Geometry: final body of the model. Coordinates: model frame, mm. Face numbers are marked on the shaded views. Give positions to 0.01 mm unless a question says otherwise; leave off trailing zeros. Write each loop counter-clockwise with the first axis right and the second up, starting at its lowest first coordinate (ties: lowest second). Pieces come first, ordered by that corner, then holes. Notation, with made-up numbers: (-15.75, 54.25) -> (30.25, 54.25) arc R19 ccw to (30.25, 64.25) -> close; hole circle Ø3 at (29.5, -11). An arc over 180 degrees is marked (long way). Answer as a JSON object with one key per item and string values.
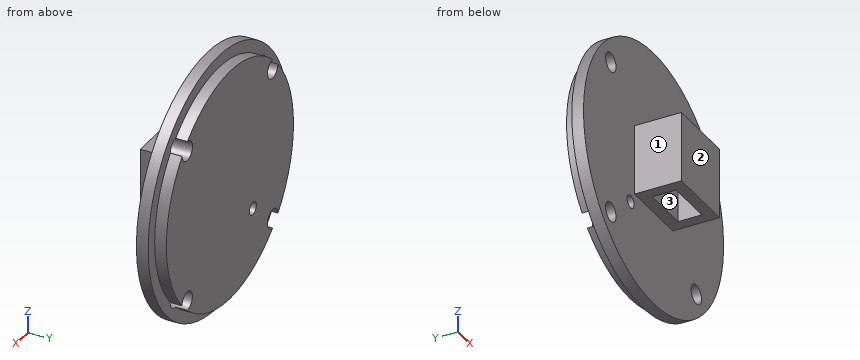
from build123d import *

# Parameters (mm, degrees)
SKETCH_1_R          = 55
EXTRUDE_1_DEPTH     = 5
SKETCH_2_R          = 49.9
EXTRUDE_2_DEPTH     = 5
SKETCH_3_W          = 30
SKETCH_3_H          = 30
EXTRUDE_3_DEPTH     = 20
SKETCH_4_W          = 20.2
SKETCH_4_H          = 10.2
CUT_EXTRUDE_1_DEPTH = 71
SKETCH_5_R          = 4.1
CUT_EXTRUDE_2_DEPTH = 11
SKETCH_6_R          = 2.75
CUT_EXTRUDE_3_DEPTH = 31


with BuildPart() as part:
    # Эскиз1 → Бобышка-Вытянуть1 (new body)
    with BuildSketch(Plane(origin=(0, 0, 0), x_dir=(1, 0, 0), z_dir=(0, 1, 0))):
        with Locations(Location((0, 0, 0), (0, 0, 270))):  # turned: the seam where the file's is
            Circle(SKETCH_1_R)
    extrude(amount=EXTRUDE_1_DEPTH)

    # Эскиз2 → Бобышка-Вытянуть2 (add)
    with BuildSketch(Plane(origin=(0, 5, 0), x_dir=(1, 0, 0), z_dir=(0, 1, 0))):
        with Locations(Location((0, 0, 0), (0, 0, 270))):  # turned: the seam where the file's is
            Circle(SKETCH_2_R)
    extrude(amount=EXTRUDE_2_DEPTH)

    # Эскиз3 → Бобышка-Вытянуть3 (add)
    with BuildSketch(Plane.XZ):
        Rectangle(SKETCH_3_W, SKETCH_3_H)
    extrude(amount=EXTRUDE_3_DEPTH)

    # Эскиз4 → Вырез-Вытянуть1 (cut, through all)
    with BuildSketch(Plane.XY.offset(15)):
        with Locations((0, -10)):
            Rectangle(SKETCH_4_W, SKETCH_4_H)
    extrude(amount=-CUT_EXTRUDE_1_DEPTH, mode=Mode.SUBTRACT)

    # Эскиз5 → Вырез-Вытянуть2 (cut, through all)
    with BuildSketch(Plane.XZ):
        with Locations(Location((33.592198598, -32.871936263, 0), (0, 0, 270))):  # turned: the seam where the file's is
            Circle(SKETCH_5_R)
        with Locations(Location((-33.591727056, -32.872418125, 0), (0, 0, 270))):  # turned: the seam where the file's is
            Circle(SKETCH_5_R)
        with Locations(Location((-33.591727056, 32.872418125, 0), (0, 0, 270))):  # turned: the seam where the file's is
            Circle(SKETCH_5_R)
        with Locations(Location((33.483215177, 32.983215177, 0), (0, 0, 270))):  # turned: the seam where the file's is
            Circle(SKETCH_5_R)
    extrude(amount=-CUT_EXTRUDE_2_DEPTH, mode=Mode.SUBTRACT)

    # Эскиз6 → Вырез-Вытянуть3 (cut, through all)
    with BuildSketch(Plane(origin=(0, 10, 0), x_dir=(1, 0, 0), z_dir=(0, 1, 0))):
        with Locations(Location((-17.999856554, 19.999999999, 0), (0, 0, 270))):  # turned: the seam where the file's is
            Circle(SKETCH_6_R)
    extrude(amount=-CUT_EXTRUDE_3_DEPTH, mode=Mode.SUBTRACT)


solid = part.part
Q1. Cut plane C-C (x = 0). Return the cut outline in (y, z), and give its area (3 significant figures).
Values:
{"outline": "(-20, -15) -> (-15.1, -15) -> (-15.1, 15) -> (-20, 15) -> close; (-4.9, -15) -> (0, -15) -> (0, -55) -> (5, -55) -> (5, -49.9) -> (10, -49.9) -> (10, 49.9) -> (5, 49.9) -> (5, 55) -> (0, 55) -> (0, 15) -> (-4.9, 15) -> close", "area": "1,340 mm²"}
Q2. First-contact query: P1, Ø6.5, axis at x = 33.59, z = -32.87, coming from the +Y side; P2, Ø3, axis at y = -10.5, z = 4, coming from the +X side; P3, Ø9, axis at x = -18, z = -20, coming from the +Y side; P4, Ø1.5, axis at x = -13, y = -6, coming from the +Z side. Flat tips, straight axial feed; report the tip coordinate or a pass-through.
Values:
{"P1": "through", "P2": "x = 15", "P3": "y = 10", "P4": "z = 15"}
Q3. Cut plane A-A (z = 0). Return the cut outline in (x, y), and give its area (3 significant figures).
Values:
{"outline": "(-55, 0) -> (-15, 0) -> (-15, -20) -> (15, -20) -> (15, 0) -> (55, 0) -> (55, 5) -> (49.9, 5) -> (49.9, 10) -> (-49.9, 10) -> (-49.9, 5) -> (-55, 5) -> close; hole (-10.1, -15.1) -> (10.1, -15.1) -> (10.1, -4.9) -> (-10.1, -4.9) -> close", "area": "1,440 mm²"}
Q4. Material intervals for L1, parallel to Y at x = 4.5, z = -6; L2, parallel to Z at x = 37, y = 3.25; L3, parallel to X at y = -10, z = 14.5, sorted ascending. Write a range as from..to.
Values:
{"L1": "-20..-15.1, -4.9..10", "L2": "-40.69..-35.15, -30.59..30.88, 35.09..40.69", "L3": "-15..-10.1, 10.1..15"}
Q5. Cut plane D-D (z = -20). Return the cut outline in (x, y), and give its area (3 significant figures).
Values:
{"outline": "(-51.23, 0) -> (-20.75, 0) -> (-20.75, 10) -> (-45.72, 10) -> (-45.72, 5) -> (-51.23, 5) -> close; (-15.25, 0) -> (51.23, 0) -> (51.23, 5) -> (45.72, 5) -> (45.72, 10) -> (-15.25, 10) -> close", "area": "915 mm²"}
Q6. Mould query, pull axis Y, two halves, no side actions, for the marked faces 1, 2 and 3. Classes: pulls with the +Y half, pulls with the -Y half, needs draft (parallel to the pull), parting line crosses it, or undercut.
Values:
{"face 1": "needs draft", "face 2": "pulls with the -Y half", "face 3": "undercut"}
Q7. Cut plane B-B (y = -10). Return the cut outline in (x, z).
Values:
{"outline": "(-15, -15) -> (-10.1, -15) -> (-10.1, 15) -> (-15, 15) -> close; (10.1, -15) -> (15, -15) -> (15, 15) -> (10.1, 15) -> close"}
